from build123d import *

# Parameters (mm, degrees)
SKETCH1_R           = 2
BOSS_EXTRUDE2_DEPTH = 2


with BuildPart() as part:
    # Sketch1 → Boss-Extrude2 (new body)
    with BuildSketch(Plane(origin=(0, 0, 0), x_dir=(1, 0, 0), z_dir=(0, 1, 0))):
        with BuildLine():
            Line((0, 48.412862342), (0, 37.692030173))
            ThreePointArc((0, 37.692030173), (0.292893219, 36.984923392), (1, 36.692030173))
            Line((1, 36.692030173), (31.48, 36.692030173))
            Line((31.48, 36.692030173), (43.036527631, 36.692030173))
            Line((43.036527631, 36.692030173), (43.036527631, 25.986950269))
            Line((43.036527631, 25.986950269), (43.036527631, 17.132198258))
            Line((43.036527631, 17.132198258), (43.036527631, 13.116497362))
            Line((43.036527631, 13.116497362), (38.310297741, 9.113727486))
            Line((38.310297741, 9.113727486), (34.253582629, 9.113727486))
            Line((34.253582629, 9.113727486), (36, 7.157074844))
            Line((36, 7.157074844), (30.071702425, 2.136241855))
            Line((30.071702425, 2.136241855), (54.200832168, 13.821577266))
            Line((54.200832168, 13.821577266), (54.200832168, 36.692030173))
            Line((54.200832168, 36.692030173), (54.200832168, 49.412862342))
            Line((54.200832168, 49.412862342), (41.48, 49.412862342))
            Line((41.48, 49.412862342), (1, 49.412862342))
            ThreePointArc((1, 49.412862342), (0.292893219, 49.119969123), (0, 48.412862342))
        make_face()
        with Locations((45.48, 41.700609081)):
            Circle(SKETCH1_R, mode=Mode.SUBTRACT)
        with BuildLine():
            Line((15, 43.700609081), (4.549516448, 43.700609081))
            Line((4.549516448, 43.700609081), (4.549516448, 39.700609081))
            Line((4.549516448, 39.700609081), (15, 39.700609081))
            ThreePointArc((15, 39.700609081), (17, 41.700609081), (15, 43.700609081))
        make_face(mode=Mode.SUBTRACT)
    extrude(amount=BOSS_EXTRUDE2_DEPTH)


solid = part.part
Model file for the job. Use its own axes, mm. A direction names the side the tool comes from. Coordinates: 2 decimals unless noted, no trailing zeros. Order: outer loops, then holes, each group sorted by start corner. A loop starts at its lowest first (then second) coordinate and runs counter-clockwise, first axis right, second up. Notation, with made-up numbers: (47.25, 30.5) -> (83.25, 30.5) arc R18 ccw to (83.25, 37.5) -> close; hole circle Ø9 at (85.5, -35). An arc over 180 degrees is marked (long way). Return JSON: item names as keys, results as strings. Group by question number.
Item 1: Saw through at C-C on y = 1.45. Write the cut outline in (x, z).
Item 2: Saw through at A-A on x = 11. Write the cut outline in (y, z), then the cut area to 3 significant figures.
Item 3: Saw through at B-B on z = -42.5. Write the cut outline in (x, y).
Item 4: Pull direction Z, two halves, no side cores. Call faces 4 (the flat face through (28, 1, -49.413)), 5 (the flat face through (0, 1, -43)), 6 (the flat face through (4.55, 1, -42)): pulls with the +Z half, pulls with the -Z half, needs draft (parallel to the pull), parting line crosses it, or undercut.
Item 5: Saw through at D-D on x = 45. Write the cut outline in (y, z).
Item 6: Tool access for faces 1 (the flat face through (35.115, 0.986, -8.149)), 2 (the cylindrical face through (17, 1, -41.7)), 3 (the flat face through (41.97, 0.99, -7.9)): list every direction of +Z, -Z, +X, -X, +Y, -Y with a clear straight run to the whole face (end or side of a thin tool).
Item 7: Wall check: line 1 along Z through (x, y) = (35.5, 1.6); line 2 along Z through (x, y) = (7, 0.1); line 3 along X through (y, z) = (0.4, -33). Give the ranges that are in metal, low to high. Write a range as [from, to].
Values found:
{
 "1": {"outline": "(0, -48.41) arc R1 ccw to (1, -49.41) -> (54.2, -49.41) -> (54.2, -13.82) -> (30.07, -2.14) -> (36, -7.16) -> (34.25, -9.11) -> (38.31, -9.11) -> (43.04, -13.12) -> (43.04, -36.69) -> (1, -36.69) arc R1 ccw to (0, -37.69) -> close; hole (4.55, -43.7) -> (15, -43.7) arc R2 ccw to (15, -39.7) -> (4.55, -39.7) -> close; hole circle Ø4 at (45.48, -41.7)"},
 "2": {"outline": "(0, -49.41) -> (2, -49.41) -> (2, -43.7) -> (0, -43.7) -> close; (0, -39.7) -> (2, -39.7) -> (2, -36.69) -> (0, -36.69) -> close", "area": "17.4 mm2"},
 "3": {"outline": "(0, 0) -> (4.55, 0) -> (4.55, 2) -> (0, 2) -> close; (16.83, 0) -> (43.65, 0) -> (43.65, 2) -> (16.83, 2) -> close; (47.31, 0) -> (54.2, 0) -> (54.2, 2) -> (47.31, 2) -> close"},
 "4": {"face 4": "pulls with the -Z half", "face 5": "needs draft", "face 6": "undercut"},
 "5": {"outline": "(0, -49.41) -> (2, -49.41) -> (2, -43.64) -> (0, -43.64) -> close; (0, -39.76) -> (2, -39.76) -> (2, -9.37) -> (0, -9.37) -> close"},
 "6": {"face 1": "-X, +Y, -Y", "face 2": "+Y, -Y", "face 3": "+Z, +X, +Y, -Y"},
 "7": {"line 1": "z = [-49.41, -36.69], [-9.11, -7.72], [-6.73, -4.77]", "line 2": "z = [-49.41, -43.7], [-39.7, -36.69]", "line 3": "x = [43.04, 54.2]"}
}
